Source: three-view drawing plus pictorial views. Frame: mm from the lowest corner of the part. Round coordinates to 2 decimals unless told otherwise and drop trailing zeros. Write each loop counter-clockwise with the first axis right and the second up, starting at its lowest first coordinate (ties: lowest second). Pieces come first, ordered by that corner, then holes. Notation, with made-up numbers: M 15,82 L 32,82 A23 cw 32,118 Z; hole C 48,-12.5 d10. An arc over 180 degrees is marked long. Put each result on its own line as item: value. Start each with the question number.
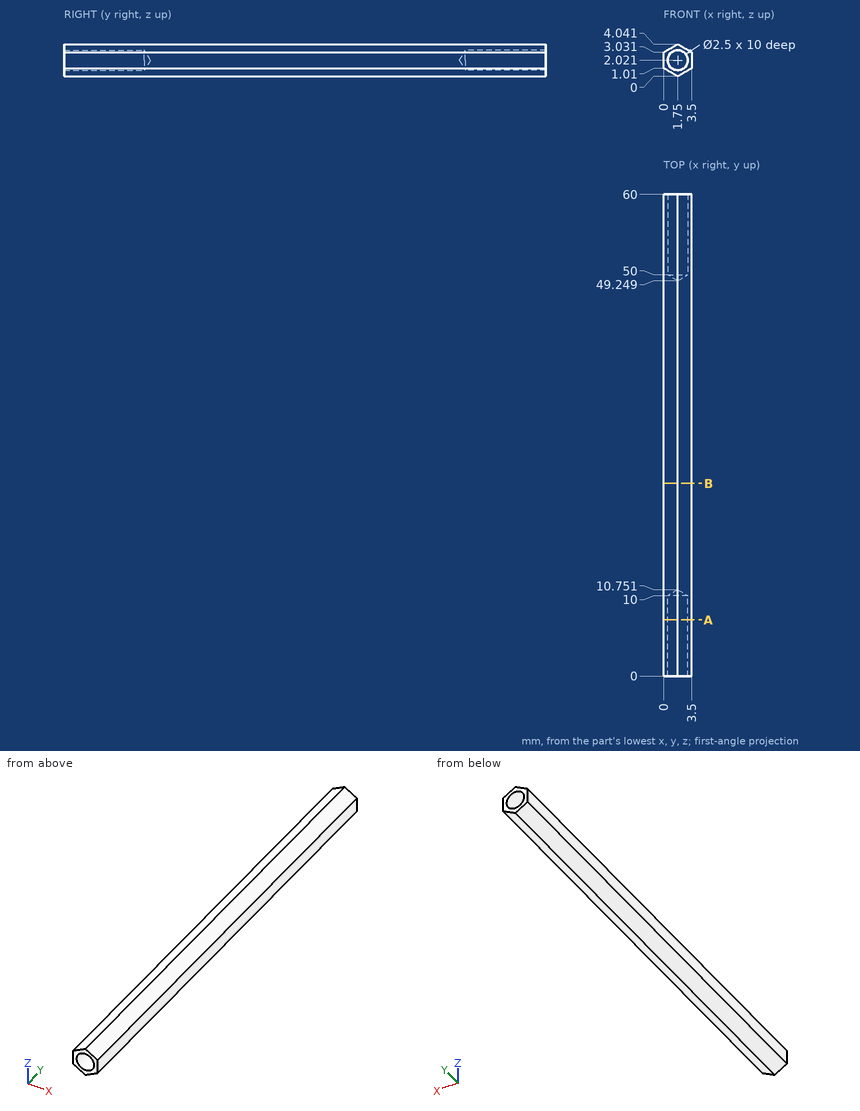
(1) Section query B-B (y = 24). Return loops of the section in (x, z), and give its area (3 significant figures).
(2) Contact query for flat-ended pins moving along their axis: P1, Ø1.5, axis at x = 1.75, z = 2.02, coming from the +Y side; P2, Ø1, axis at x = 1.5, z = 1, coming from the -Y side. Output: stop coordinate, or through.
(3) Section query A-A (y = 7). Return loops of the section in (x, z).
(4) Ray query, line 1 along Z through (x, y) = (1.75, 7); line 2 along Z through (x, y) = (1.15, 55) (1 decimal); line 3 along X through (y, z) = (53.5, 2.7). Return the intervals inside material, ascending.
Entries:
1. outline: M 0,1.01 L 1.75,0 L 3.5,1.01 L 3.5,3.03 L 1.75,4.04 L 0,3.03 Z
1. area: 10.6 mm2
2. P1: y = 49.7
2. P2: y = 0
3. outline: M 0,1.01 L 1.75,0 L 3.5,1.01 L 3.5,3.03 L 1.75,4.04 L 0,3.03 Z; hole C 1.75,2.02 d2.5
4. line 1: 0 to 0.77, 3.27 to 4.04
4. line 2: 0.3 to 0.9, 3.1 to 3.7
4. line 3: 0 to 0.7, 2.8 to 3.5
